The model under review builds one solid part; all positions refer to its coordinate system, in mm. Face numbers are marked on the shaded views. A direction names the side the tool comes from. Coordinates: 2 decimals unless noted, no trailing zeros. Order: outer loops, then holes, each group sorted by start corner. A loop starts at its lowest first (then second) coordinate and runs counter-clockwise, first axis right, second up.
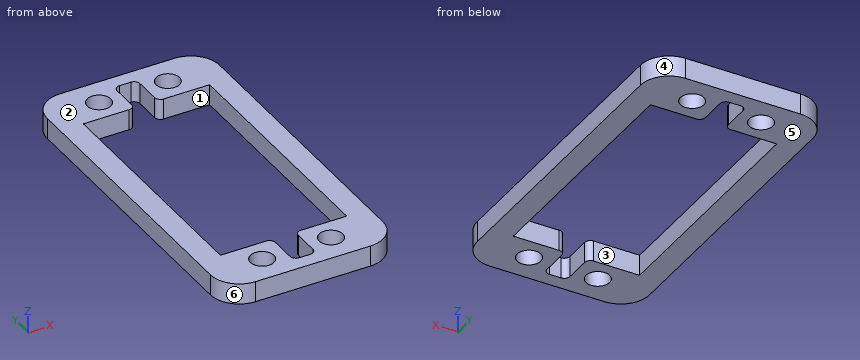
```python
from build123d import *

# Parameters (mm, degrees)
CROQUIS1_W              = 30
CROQUIS1_H              = 60
SALIENTE_EXTRUIR1_DEPTH = 3.62
CROQUIS2_W              = 22
CROQUIS2_H              = 42
CORTAR_EXTRUIR1_DEPTH   = 34.73580294
CROQUIS3_R              = 2.05
CORTAR_EXTRUIR2_DEPTH   = 34.73580294
REDONDEO1_R             = 5
REDONDEO3_R             = 1


with BuildPart() as part:
    # Croquis1 → Saliente-Extruir1 (new body)
    with BuildSketch(Plane.XY):
        Rectangle(CROQUIS1_W, CROQUIS1_H)
    extrude(amount=SALIENTE_EXTRUIR1_DEPTH)

    # Croquis2 → Cortar-Extruir1 (cut, through all)
    with BuildSketch(Plane(origin=(0, 0, 0), x_dir=(-1, 0, 0), z_dir=(0, 0, -1))):
        Rectangle(CROQUIS2_W, CROQUIS2_H)
    extrude(amount=-CORTAR_EXTRUIR1_DEPTH, mode=Mode.SUBTRACT)

    # Croquis3 → Cortar-Extruir2 (cut, through all)
    with BuildSketch(Plane(origin=(0, 0, 0), x_dir=(-1, 0, 0), z_dir=(0, 0, -1))):
        with Locations((-6, 25)):
            Circle(CROQUIS3_R)
        with Locations((6, 25)):
            Circle(CROQUIS3_R)
        with Locations((-6, -25)):
            Circle(CROQUIS3_R)
        with Locations((6, -25)):
            Circle(CROQUIS3_R)
        Polygon((-2, 21), (-2, 27.5), (2, 27.5), (2, -27.5), (-2, -27.5), align=None)
    extrude(amount=-CORTAR_EXTRUIR2_DEPTH, mode=Mode.SUBTRACT)

    # Redondeo1
    redondeo1_edges = [part.edges().sort_by_distance(p)[0] for p in [
        (-15, 30, 1.81),
        (15, 30, 1.81),
        (15, -30, 1.81),
        (-15, -30, 1.81),
    ]]
    fillet(redondeo1_edges, radius=REDONDEO1_R)

    # Redondeo3
    redondeo3_edges = [part.edges().sort_by_distance(p)[0] for p in [
        (2, -21, 1.81),
        (-2, -21, 1.81),
        (-2, 21, 1.81),
        (-2, 27.5, 1.81),
        (2, 21, 1.81),
        (2, -27.5, 1.81),
        (-2, -27.5, 1.81),
        (2, 27.5, 1.81),
    ]]
    fillet(redondeo3_edges, radius=REDONDEO3_R)


solid = part.part
```
(1) We need section D-D, the plane x = -6.75. Write out the cut boundary in (y, z), and give its area (3 significant figures).
A:
outline: (-30, 0) - (-26.91, 0) - (-26.91, 3.62) - (-30, 3.62) - close; (-23.09, 0) - (-21, 0) - (-21, 3.62) - (-23.09, 3.62) - close; (21, 0) - (23.09, 0) - (23.09, 3.62) - (21, 3.62) - close; (26.91, 0) - (30, 0) - (30, 3.62) - (26.91, 3.62) - close
area: 37.5 mm2
(2) We need section C-C, the plane z = 2.35. Count the separate pieces of the cut face and the enclosed holes in it, and give its area (3 significant figures).
A:
separate pieces: 1
enclosed holes: 5
area: 750 mm2
(3) For pin 1 Ø1.8 at (y, z) = (25.5, 2.5) entering from -X, flat-tipped, find the tip position at first contact; note if it passes through.
A:
pin 1: stops at x = -15
(4) Wall thickness on probe 1 along Y at (x, z) = (-6, 2.4); probe 2 along X at (y, z) = (-11.5, 0.6); probe 3 along Y at (x, z) = (-3.5, 0.3): over which ranges is each line inside the solid? List them lowest first.
A:
probe 1: y = -30 to -27.05, -22.95 to -21, 21 to 22.95, 27.05 to 30
probe 2: x = -15 to -11, 11 to 15
probe 3: y = -30 to -21, 21 to 30
(5) Machinability: for the marked faces 1 and 2, which of the approach directions +Z, -Z, +X, -X, +Y, -Y give a long, thin tool a straight path to every point of the face, cutting with its end or side? Answer none if there is none.
A:
face 1: +Z, -Z
face 2: +Z, +X, -X, +Y, -Y
(6) We need section A-A, the plane x = 6. Write out the cut boundary in (y, z).
A:
outline: (-30, 0) - (-27.05, 0) - (-27.05, 3.62) - (-30, 3.62) - close; (-22.95, 0) - (-21, 0) - (-21, 3.62) - (-22.95, 3.62) - close; (21, 0) - (22.95, 0) - (22.95, 3.62) - (21, 3.62) - close; (27.05, 0) - (30, 0) - (30, 3.62) - (27.05, 3.62) - close
(7) We need section B-B, the plane y = -2.5. Write out the cut boundary in (x, z).
A:
outline: (-15, 0) - (-11, 0) - (-11, 3.62) - (-15, 3.62) - close; (11, 0) - (15, 0) - (15, 3.62) - (11, 3.62) - close
(8) Draft analysis for pull direction Y (two halves, no side actions). For the marked faces 3, 4, 5 and 6, state which applies: released by +Y, released by -Y, zero draft, split by the parting line, or undercut.
A:
face 3: undercut
face 4: released by +Y
face 5: zero draft
face 6: released by -Y
